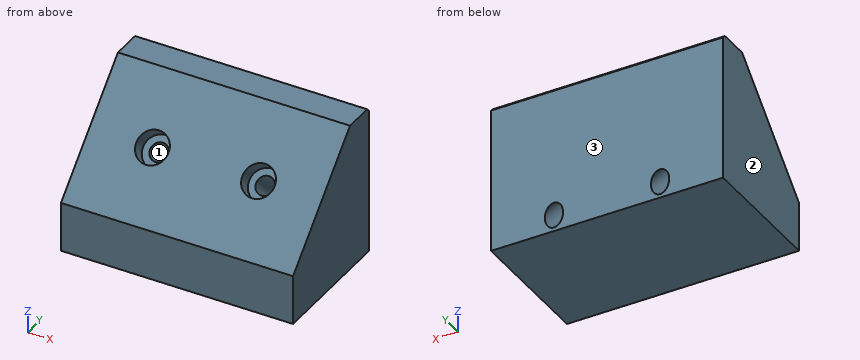
```python
from build123d import *

# Parameters (mm, degrees)
F0_W           = 70
F0_H           = 40
F1_DEPTH       = 45
F2_SIZE        = 30
F4_D           = 5.5
F4_CBORE_D     = 9.75
F4_CBORE_DEPTH = 5
F5_SIZE        = 1


with BuildPart() as f1:
    # F0 (on Top) → F1 (new body)
    with BuildSketch(Plane.XY):
        with Locations((-66.7884647846, -34.8549866823)):
            Rectangle(F0_W, F0_H)
    extrude(amount=F1_DEPTH)

    # F2
    f2_edges = [f1.edges().sort_by_distance(p)[0] for p in [
        (-66.788465, -54.854987, 45),
    ]]
    chamfer(f2_edges, length=F2_SIZE)

    # F4 (through all)
    with Locations(Plane(origin=(0, -34.9274933411, 34.9274933411), x_dir=(1, 0, 0), z_dir=(0, -0.7071067812, 0.7071067812))):
        with Locations((-82.7884647846, -6.9685279115), (-50.7884647846, -6.9685279115)):
            CounterBoreHole(F4_D / 2, F4_CBORE_D / 2, F4_CBORE_DEPTH)

    # F5
    f5_edges = [f1.edges().sort_by_distance(p)[0] for p in [
        (-66.788465, -14.854987, 45),
    ]]
    chamfer(f5_edges, length=F5_SIZE)


solid = f1.part
```
Read the model definition and answer for the solid it produces. Units are mm, in the model's axes. Face numbers are marked on the shaded views. Give positions to 0.01 mm unless a question says otherwise; leave off trailing zeros. Loops run counter-clockwise (first coordinate to the right, second up) from the corner with the lowest first, then second, coordinate; pieces in that order, holes last.
Item 1: The mould has two halves that part along Y. Classify the marked faces 1, 2 and 3: released by +Y, released by -Y, zero draft, split by the parting line, or undercut.
Item 2: The part is cut by section C-C (z = 40). Write down the section's boundary in (x, y), and give its area (3 significant figures).
Item 3: Each of these flat-tipped pins is pushed along its axis until it touches: pin 1 Ø10 at (x, y) = (-58, -32) entering from +Z (3 decimals); pin 2 Ø8 at (x, z) = (-58.5, 23) entering from -Y (3 decimals). Where does it stop, or does it pass through?
Item 4: Find the intervals of material crossed by line 1 along X through (y, z) = (-34, 21); line 2 along Y through (x, z) = (-52.5, 26); line 3 along Z through (x, y) = (-48.5, -21), in increasing order.
Item 5: The part is cut by section A-A (x = -81). Write down the section's boundary in (y, z), and give its area (3 significant figures).
Item 6: The part is cut by section D-D (y = -29). Give the number of separate pieces and of enclosed holes in the cut face, and give its area (3 significant figures).
Item 7: The part is cut by section B-B (x = -64). Write down the section's boundary in (y, z), and give its area (3 significant figures).
Taken from the geometry:
1. face 1: undercut
1. face 2: zero draft
1. face 3: released by +Y
2. outline: (-101.79, -29.85) - (-31.79, -29.85) - (-31.79, -14.85) - (-101.79, -14.85) - close
2. area: 1,050 mm2
3. pin 1: stops at z = 42.855
3. pin 2: stops at y = -50.855
4. line 1: x = -101.79 to -84.41, -81.17 to -52.41, -49.17 to -31.79
4. line 2: y = -43.85 to -42.31, -32.81 to -14.85
4. line 3: z = 0 to 8.99, 13.3 to 45
5. outline: (-54.85, 0) - (-14.85, 0) - (-14.85, 2.05) - (-37.8, 24.99) - (-39.53, 23.26) - (-43.06, 26.79) - (-54.85, 15) - close; (-36.65, 33.21) - (-33.11, 29.67) - (-34.84, 27.94) - (-14.85, 7.95) - (-14.85, 44) - (-15.85, 45) - (-24.85, 45) - close
5. area: 1,180 mm2
6. separate pieces: 1
6. enclosed holes: 2
6. area: 2,790 mm2
7. outline: (-54.85, 0) - (-14.85, 0) - (-14.85, 44) - (-15.85, 45) - (-24.85, 45) - (-54.85, 15) - close
7. area: 1,350 mm2
